CAD build for the part. Positions are in the model's coordinates, mm. Coordinates: 2 decimals unless noted, no trailing zeros. Write item = value, one per line.
from build123d import *

# Parameters (mm, degrees)
SKETCH1_W           = 450.2
SKETCH1_H           = 228.6
BOSS_EXTRUDE1_DEPTH = 6.35
CORNER_SLOTS_DEPTH  = 10
FOOT_HOLES_1_4_20_D = 8.7376
ESD_FASTERNERS_D    = 4.7625
MIDDLE_SLOTS_DEPTH  = 10


with BuildPart() as part:
    # Sketch1 → Boss-Extrude1 (new body)
    with BuildSketch(Plane.XY):
        Rectangle(SKETCH1_W, SKETCH1_H)
    extrude(amount=BOSS_EXTRUDE1_DEPTH)

    # Sketch3 → Corner Slots (cut)
    with BuildSketch(Plane.XY.offset(6.35)):
        with BuildLine():
            ThreePointArc((-180.908290444, 58.084863229), (-180.908290444, 60.913290444), (-178.079863229, 60.913290444))
            Line((-178.079863229, 60.913290444), (-172.691709556, 55.525136771))
            ThreePointArc((-172.691709556, 55.525136771), (-172.691709556, 52.696709556), (-175.520136771, 52.696709556))
            Line((-175.520136771, 52.696709556), (-180.908290444, 58.084863229))
        make_face()
        with BuildLine():
            ThreePointArc((-184.500392892, 67.333820108), (-184.500392892, 64.505392892), (-187.328820108, 64.505392892))
            Line((-187.328820108, 64.505392892), (-192.71697378, 69.893546565))
            ThreePointArc((-192.71697378, 69.893546565), (-192.71697378, 72.72197378), (-189.888546565, 72.72197378))
            Line((-189.888546565, 72.72197378), (-184.500392892, 67.333820108))
        make_face()
        with BuildLine():
            Line((189.888546565, 72.72197378), (184.500392892, 67.333820108))
            ThreePointArc((184.500392892, 67.333820108), (184.500392892, 64.505392892), (187.328820108, 64.505392892))
            Line((187.328820108, 64.505392892), (192.71697378, 69.893546565))
            ThreePointArc((192.71697378, 69.893546565), (192.71697378, 72.72197378), (189.888546565, 72.72197378))
        make_face()
        with BuildLine():
            Line((175.520136771, 52.696709556), (180.908290444, 58.084863229))
            ThreePointArc((180.908290444, 58.084863229), (180.908290444, 60.913290444), (178.079863229, 60.913290444))
            Line((178.079863229, 60.913290444), (172.691709556, 55.525136771))
            ThreePointArc((172.691709556, 55.525136771), (172.691709556, 52.696709556), (175.520136771, 52.696709556))
        make_face()
        with BuildLine():
            ThreePointArc((184.500392892, -67.333820108), (184.500392892, -64.505392892), (187.328820108, -64.505392892))
            Line((187.328820108, -64.505392892), (192.71697378, -69.893546565))
            ThreePointArc((192.71697378, -69.893546565), (192.71697378, -72.72197378), (189.888546565, -72.72197378))
            Line((189.888546565, -72.72197378), (184.500392892, -67.333820108))
        make_face()
        with BuildLine():
            ThreePointArc((180.908290444, -58.084863229), (180.908290444, -60.913290444), (178.079863229, -60.913290444))
            Line((178.079863229, -60.913290444), (172.691709556, -55.525136771))
            ThreePointArc((172.691709556, -55.525136771), (172.691709556, -52.696709556), (175.520136771, -52.696709556))
            Line((175.520136771, -52.696709556), (180.908290444, -58.084863229))
        make_face()
        with BuildLine():
            Line((-172.691709556, -55.525136771), (-178.079863229, -60.913290444))
            ThreePointArc((-178.079863229, -60.913290444), (-180.908290444, -60.913290444), (-180.908290444, -58.084863229))
            Line((-180.908290444, -58.084863229), (-175.520136771, -52.696709556))
            ThreePointArc((-175.520136771, -52.696709556), (-172.691709556, -52.696709556), (-172.691709556, -55.525136771))
        make_face()
        with BuildLine():
            Line((-189.888546565, -72.72197378), (-184.500392892, -67.333820108))
            ThreePointArc((-184.500392892, -67.333820108), (-184.500392892, -64.505392892), (-187.328820108, -64.505392892))
            Line((-187.328820108, -64.505392892), (-192.71697378, -69.893546565))
            ThreePointArc((-192.71697378, -69.893546565), (-192.71697378, -72.72197378), (-189.888546565, -72.72197378))
        make_face()
    extrude(amount=-CORNER_SLOTS_DEPTH, mode=Mode.SUBTRACT)

    # Foot Holes 1/4-20 (through all)
    with Locations(Plane.XY.offset(6.35)):
        with Locations((-212.4, 101.6), (-212.4, -101.6)):
            foot_holes_1_4_20 = Hole(FOOT_HOLES_1_4_20_D / 2)

    # Mirror2: Foot Holes 1/4-20 across plane
    add(foot_holes_1_4_20.mirror(Plane(origin=(0, 0, 0), x_dir=(0, 0, 1), z_dir=(1, 0, 0))), mode=Mode.SUBTRACT)

    # ESD Fasterners (through all)
    with Locations(Plane.XY.offset(6.35)):
        with Locations((-75.1, 99.09), (75.1, -99.089)):
            Hole(ESD_FASTERNERS_D / 2)

    # Sketch16 → Middle Slots (cut)
    with BuildSketch(Plane.XY):
        with BuildLine():
            Line((2, -78.63), (2, -86.25))
            ThreePointArc((2, -86.25), (0, -88.25), (-2, -86.25))
            Line((-2, -86.25), (-2, -78.63))
            ThreePointArc((-2, -78.63), (0, -76.63), (2, -78.63))
        make_face()
        with BuildLine():
            Line((-2, -69.55), (-2, -61.93))
            ThreePointArc((-2, -61.93), (0, -59.93), (2, -61.93))
            Line((2, -61.93), (2, -69.55))
            ThreePointArc((2, -69.55), (0, -71.55), (-2, -69.55))
        make_face()
        with BuildLine():
            Line((2, 78.63), (2, 86.25))
            ThreePointArc((2, 86.25), (0, 88.25), (-2, 86.25))
            Line((-2, 86.25), (-2, 78.63))
            ThreePointArc((-2, 78.63), (0, 76.63), (2, 78.63))
        make_face()
        with BuildLine():
            Line((-2, 69.55), (-2, 61.93))
            ThreePointArc((-2, 61.93), (0, 59.93), (2, 61.93))
            Line((2, 61.93), (2, 69.55))
            ThreePointArc((2, 69.55), (0, 71.55), (-2, 69.55))
        make_face()
    extrude(amount=MIDDLE_SLOTS_DEPTH, mode=Mode.SUBTRACT)


solid = part.part
(1) Pin check, flat tip, straight feed: pin 1 Ø7 at (x, y) = (-212.4, -101.6) entering from -Z. Stop position of the tip, or through.
Evaluation:
pin_1 = through
(2) Pull direction Y, two halves, no side cores. Call faces 1 (the face through (-211.83, -97.27, 3.13)), 2 (the face through (-3, 2, 6.35)): +Y half, -Y half, draft (parallel to the pull), parting line (faces both ways), or undercut.
Evaluation:
face_1 = undercut
face_2 = draft
(3) Wall check: line 1 (Y direction, x = -212.4, z = 5.25); line 2 (Y direction, x = 186.5, z = 4.75); line 3 (X direction, y = 71, z = 1.25). Give the ranges that are in metal, low to high. Write a range as from..to.
Evaluation:
line_1 = -114.3..-105.97, -97.23..97.23, 105.97..114.3
line_2 = -114.3..-69.33, -64.01..64.01, 69.33..114.3
line_3 = -225.1..-193.28, -188.17..-1.38, 1.38..188.17, 193.28..225.1
